```python
from build123d import *

# Parameters (mm, degrees)
EXTRUDE_1_DEPTH          = 6
SKETCH_2_W               = 218
SKETCH_2_H               = 6
EXTRUDE_2_DEPTH          = 6
CUT_EXTRUDE_5_DEPTH      = 153.515572975
CUT_EXTRUDE_5_DEPTH_BACK = 153.515572975
SKETCH_9_W               = 30
SKETCH_9_H               = 6


with BuildPart() as part:
    # Эскиз1 → Бобышка-Вытянуть1 (new body)
    with BuildSketch(Plane(origin=(0, 0, 0), x_dir=(1, 0, 0), z_dir=(0, 1, 0))):
        Polygon((26.333333333, 100), (26.333333333, 94), (2.45, 94), (2.45, 83), (3.925, 83), (3.925, 79.2), (2.45, 79.2), (2.45, 75), (-2.45, 75), (-2.45, 79.2), (-3.925, 79.2), (-3.925, 83), (-2.45, 83), (-2.45, 94), (-26.333333333, 94), (-26.333333333, 100), (-56.333333333, 100), (-56.333333333, 94), (-70.05, 94), (-70.05, 83), (-68.575, 83), (-68.575, 79.2), (-70.05, 79.2), (-70.05, 75), (-74.95, 75), (-74.95, 79.2), (-76.425, 79.2), (-76.425, 83), (-74.95, 83), (-74.95, 94), (-109, 94), (-109, 91), (-115, 91), (-115, 81), (-109, 81), (-109, 72.5875), (-98, 72.5875), (-98, 74.0625), (-94.2, 74.0625), (-94.2, 72.5875), (-90, 72.5875), (-90, 67.6875), (-94.2, 67.6875), (-94.2, 66.2125), (-98, 66.2125), (-98, 67.6875), (-109, 67.6875), (-109, 20.8625), (-115, 20.8625), (-115, 10.8625), (-109, 10.8625), (-109, 2.45), (-98, 2.45), (-98, 3.925), (-94.2, 3.925), (-94.2, 2.45), (-90, 2.45), (-90, -2.45), (-94.2, -2.45), (-94.2, -3.925), (-98, -3.925), (-98, -2.45), (-109, -2.45), (-109, -10.8625), (-115, -10.8625), (-115, -20.8625), (-109, -20.8625), (-109, -67.6875), (-98, -67.6875), (-98, -66.2125), (-94.2, -66.2125), (-94.2, -67.6875), (-90, -67.6875), (-90, -72.5875), (-94.2, -72.5875), (-94.2, -74.0625), (-98, -74.0625), (-98, -72.5875), (-109, -72.5875), (-109, -81), (-115, -81), (-115, -91), (-109, -91), (-109, -94), (109, -94), (109, -91), (115, -91), (115, -81), (109, -81), (109, -72.5875), (98, -72.5875), (98, -74.0625), (94.2, -74.0625), (94.2, -72.5875), (90, -72.5875), (90, -67.6875), (94.2, -67.6875), (94.2, -66.2125), (98, -66.2125), (98, -67.6875), (109, -67.6875), (109, -20.8625), (115, -20.8625), (115, -10.8625), (109, -10.8625), (109, -2.45), (98, -2.45), (98, -3.925), (94.2, -3.925), (94.2, -2.45), (90, -2.45), (90, 2.45), (94.2, 2.45), (94.2, 3.925), (98, 3.925), (98, 2.45), (109, 2.45), (109, 10.8625), (115, 10.8625), (115, 20.8625), (109, 20.8625), (109, 67.6875), (98, 67.6875), (98, 66.2125), (94.2, 66.2125), (94.2, 67.6875), (90, 67.6875), (90, 72.5875), (94.2, 72.5875), (94.2, 74.0625), (98, 74.0625), (98, 72.5875), (109, 72.5875), (109, 81), (115, 81), (115, 91), (109, 91), (109, 94), (74.95, 94), (74.95, 83), (76.425, 83), (76.425, 79.2), (74.95, 79.2), (74.95, 75), (70.05, 75), (70.05, 79.2), (68.575, 79.2), (68.575, 83), (70.05, 83), (70.05, 94), (56.333333333, 94), (56.333333333, 100), align=None)
    extrude(amount=EXTRUDE_1_DEPTH)

    # Эскиз2 → Бобышка-Вытянуть2 (add)
    with BuildSketch(Plane(origin=(0, 6, 0), x_dir=(1, 0, 0), z_dir=(0, 1, 0))):
        with Locations((0, -97)):
            Rectangle(SKETCH_2_W, SKETCH_2_H)
    extrude(amount=-EXTRUDE_2_DEPTH)

    # Эскиз9 → Вырез-Вытянуть5 (cut, two sides: drawn at the far end of the back side and taken through both)
    with BuildSketch(Plane(origin=(0, 6, 0), x_dir=(1, 0, 0), z_dir=(0, 1, 0)).offset(-CUT_EXTRUDE_5_DEPTH_BACK)):
        with Locations((-55, -91)):
            Rectangle(SKETCH_9_W, SKETCH_9_H)
        with Locations((55, -91)):
            Rectangle(SKETCH_9_W, SKETCH_9_H)
    extrude(amount=CUT_EXTRUDE_5_DEPTH + CUT_EXTRUDE_5_DEPTH_BACK, mode=Mode.SUBTRACT)


solid = part.part
```
Source: CAD feature listing. Evaluate the final solid. Frame: model axes, mm. A direction names the side the tool comes from. Coordinates: 2 decimals unless noted, no trailing zeros. Loops run counter-clockwise (first coordinate to the right, second up) from the corner with the lowest first, then second, coordinate; pieces in that order, holes last. Notation, with made-up numbers: M 5,79 L 38,79 A30 cw 38,112 Z; hole C 27,-32 d11. An arc over 180 degrees is marked long. Use a Markdown table: item, result. Add a question column.
Q1. Section query A-A, the plane x = 47.5. Return loops of the section in (y, z), and give its area (3 significant figures).
Q2. Section query C-C, the plane z = -59. Return loops of the section in (x, y).
Q3. Draft query along Z for faces 5 (the flat face through (70, 3, 91)), 6 (the flat face through (42, 3, -100)), 7 (the flat face through (-74.95, 3, -88)). Return one class per face: pulls with the +Z half, pulls with the -Z half, needs draft (parallel to the pull), parting line crosses it, or undercut.
Q4. Section query B-B, the plane y = 3.3. State how many separate pieces and enclosed holes the cut face has, and give its area (3 significant figures).
Q5. Material intervals for L1, parallel to X at y = 3.95, z = -85; L2, parallel to Z at x = 101, y = 4.4; L3, parallel to Z at x = 48, y = 3.75, sorted ascending.
Q6. First-contact query: pin 1 (1.6 mm diameter, centred on y = 2.5, z = 3, fed in from +X); pin 2 (2 mm diameter, centred on y = 2, z = -78, fed in from -X); pin 3 (5 mm diameter, centred on x = -34, z = 5.5, fed in from -Y). Flat tips, straight axial feed; report the tip coordinate or a pass-through.
Q7. Access query for faces 1 (the flat face through (104, 3, 2.45)), 2 (the flat face through (-90, 3, 0)), 3 (the flat face through (56.333, 3, -97)), 4 (the flat face through (15, 3, -94)). Directions: +Z, -Z, +X, -X, +Y, -Y. A direction counts if a zero-diameter tool reaches every point of the face in a straight line with its end or side. Return the directions, or none.
Result:
| question | item | result |
|---|---|---|
| 1 | outline | M 0,-100 L 6,-100 L 6,88 L 0,88 Z; M 0,94 L 6,94 L 6,100 L 0,100 Z |
| 1 | area | 1,160 mm2 |
| 2 | outline | M -109,0 L 109,0 L 109,6 L -109,6 Z |
| 3 | face 5 | undercut |
| 3 | face 6 | pulls with the -Z half |
| 3 | face 7 | needs draft |
| 4 | separate pieces | 1 |
| 4 | enclosed holes | 2 |
| 4 | area | 41,800 mm2 |
| 5 | L1 | x = -115 to -74.95, -70.05 to -2.45, 2.45 to 70.05, 74.95 to 115 |
| 5 | L2 | z = -94 to -72.59, -67.69 to -2.45, 2.45 to 67.69, 72.59 to 100 |
| 5 | L3 | z = -100 to 88, 94 to 100 |
| 6 | pin 1 | stops at x = 109 |
| 6 | pin 2 | stops at x = -109 |
| 6 | pin 3 | stops at y = 0 |
| 7 | face 1 | +X, +Y, -Y |
| 7 | face 2 | -X, +Y, -Y |
| 7 | face 3 | -Z, +X, +Y, -Y |
| 7 | face 4 | -Z, +Y, -Y |
